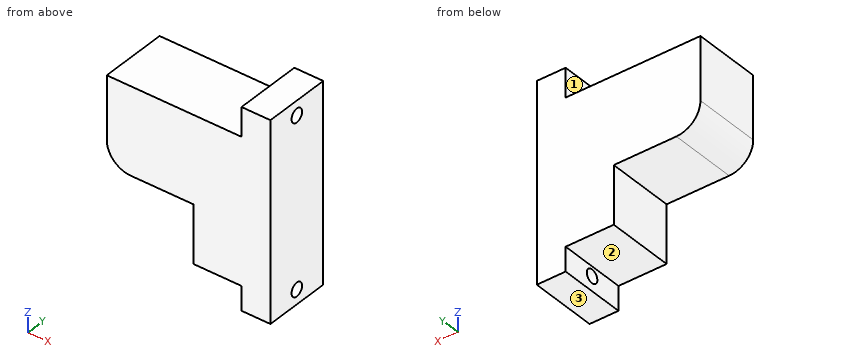
Autodesk Inventor part; units mm, degrees
ref_plane "YZ Plane" through (0, 0, 0) normal (1, 0, 0) x (0, 1, 0)
ref_plane "XZ Plane" through (0, 0, 0) normal (0, 1, 0) x (-1, 0, 0)
ref_plane "XY Plane" through (0, 0, 0) normal (0, 0, 1) x (1, 0, 0)
sketch "Sketch1" plane through (0, 0, 0) normal (1, 0, 0) x (0, 1, 0)
  line L0 (0, 0) -> (14, 0)
  line L1 (14, 0) -> (14, -30)
  line L2 (14, -30) -> (0, -30)
  line L3 (0, -30) -> (0, 0)
  line L4 (14, -30) -> (0, -30)
  line L5 (0, -30) -> (0, -30)
  line L6 (0, -30) -> (14, -30)
  line L7 (14, -30) -> (14, -30)
  line L8 (0, 0) -> (0, -18)
  line L9 (0, -18) -> (14, -18)
  line L10 (14, -18) -> (14, 0)
  point P0 (14, -18)
  dimension "d12" = 14
  dimension "d13" = 30
  dimension "d14" = 12
  dimension "d15" = 0
extrude "Extrusion6" add sketch "Sketch1" along normal blind 10 contours L9 L1 L2 L3
extrude "Extrusion7" add sketch "Sketch1" along normal blind 10 and the other way blind 18 contours L0 L1 L9 L3
fillet "Fillet2" radius 5 1 edges at (-18, 7, -18)
sketch "Sketch7" plane through (10, 0, 0) normal (1, 0, 0) x (0, 0, -1)
  line L0 (35, 14) -> (-6, 14)
  line L1 (-6, 14) -> (-6, 0)
  line L2 (-6, 0) -> (35, 0)
  line L3 (35, 0) -> (35, 14)
  line L4 (30, 0) -> (30, 14)
  circle A0 centre (32, 7) radius 1.4
  circle A1 centre (-3, 7) radius 1.4
  point P0 (0, 0)
  dimension "d32" = 41
  dimension "d33" = 5
  dimension "d34" = 14
  dimension "d35" = 2.8
  dimension "d36" = 3
  dimension "d37" = 2.8
  dimension "d38" = 35
extrude "Extrusion9" add sketch "Sketch7" along normal blind 6
properties part number "_3DPrint"
CAD build for the part. Positions are in the model's coordinates, mm. Face numbers are marked on the shaded views. A direction names the side the tool comes from. Give positions to 0.01 mm unless a question says otherwise; leave off trailing zeros. Loops run counter-clockwise (first coordinate to the right, second up) from the corner with the lowest first, then second, coordinate; pieces in that order, holes last. Notation, with made-up numbers: (5, 17) -> (23, 17) arc R13 cw to (23, 33) -> close; hole circle Ø11 at (88, 32). An arc over 180 degrees is marked (long way). Use a Markdown table: item, result.
1. Wall check: L1, parallel to Y at x = 14.05, z = 3; L2, parallel to X at y = 12, z = -26; L3, parallel to X at y = 12.5, z = 4. Give the ranges that are in metal, low to high. Write a range as [from, to].
Check result:
| item | result |
|---|---|
| L1 | y = [0, 5.6], [8.4, 14] |
| L2 | x = [0, 16] |
| L3 | x = [10, 16] |
2. Flat gauge pins, fed straight in: pin 1 (2 mm diameter, centred on x = -4.5, y = 10, fed in from -Z); pin 2 (1.8 mm diameter, centred on y = 4.5, z = 2.5, fed in from -X); pin 3 (6 mm diameter, centred on y = 4, z = -22, fed in from -X); pin 4 (6 mm diameter, centred on x = 9.5, y = 9, fed in from -Z). Where does each tip first touch, or does it go through?
Check result:
| item | result |
|---|---|
| pin 1 | stops at z = -18 |
| pin 2 | stops at x = 10 |
| pin 3 | stops at x = 0 |
| pin 4 | stops at z = -35 |
3. Slice it at B-B (z = 3). List the corners of the cut face in (x, y), plus the area to 3 significant figures.
Check result:
| item | result |
|---|---|
| outline | (10, 0) -> (16, 0) -> (16, 5.6) -> (10, 5.6) -> close; (10, 8.4) -> (16, 8.4) -> (16, 14) -> (10, 14) -> close |
| area | 67.2 mm^2 |
4. Slice it at C-C (y = 12). List the corners of the cut face in (x, z), plus the area to 3 significant figures.
Check result:
| item | result |
|---|---|
| outline | (-18, -13) arc R5 ccw to (-13, -18) -> (0, -18) -> (0, -30) -> (10, -30) -> (10, -35) -> (16, -35) -> (16, 6) -> (10, 6) -> (10, 0) -> (-18, 0) -> close |
| area | 865 mm^2 |
5. Slice it at D-D (x = 3.5). List the corners of the cut face in (y, z), plus the area to 3 significant figures.
Check result:
| item | result |
|---|---|
| outline | (0, -30) -> (14, -30) -> (14, 0) -> (0, 0) -> close |
| area | 420 mm^2 |
6. Which spindle directions (+Z, -Z, +X, -X, +Y, -Y) get a long thin tool onto all of the face, cutting with end or side? Do the marked faces 1, 2 and 3. Say none if no direction does.
Check result:
| item | result |
|---|---|
| face 1 | +Z, -X, +Y, -Y |
| face 2 | -Z, -X, +Y, -Y |
| face 3 | -Z, +X, -X, +Y, -Y |
7. Slice it at A-A (y = 7). List the corners of the cut face in (x, z), plus the area to 3 significant figures.
Check result:
| item | result |
|---|---|
| outline | (-18, -13) arc R5 ccw to (-13, -18) -> (0, -18) -> (0, -30) -> (10, -30) -> (10, -30.6) -> (16, -30.6) -> (16, 1.6) -> (10, 1.6) -> (10, 0) -> (-18, 0) -> close; (10, -35) -> (16, -35) -> (16, -33.4) -> (10, -33.4) -> close; (10, 4.4) -> (16, 4.4) -> (16, 6) -> (10, 6) -> close |
| area | 831 mm^2 |
